CAD build for the part. Positions are in the model's coordinates, mm. A direction names the side the tool comes from. Coordinates: 2 decimals unless noted, no trailing zeros. Order: outer loops, then holes, each group sorted by start corner. A loop starts at its lowest first (then second) coordinate and runs counter-clockwise, first axis right, second up. Notation, with made-up numbers: (54.5, 0.25) - (107.5, 0.25) arc R15 cw to (107.5, 8.25) - close; hole circle Ø10 at (3.5, -28). An arc over 180 degrees is marked (long way). Use one line per item in the form item = value.
```python
from build123d import *

# Parameters (mm, degrees)
F0_R          = 12.7
F1_DEPTH      = 419.1
F0_W          = 165.1
F0_H          = 152.4
F2_DEPTH      = 685.8
F3_DEPTH      = 25.4
F8_DEPTH      = 165.1010001
F8_DEPTH_BACK = 165.1010001
F9_R          = 25.4


with BuildPart() as f1:
    # F0 (on Top) → F1 (new body)
    with BuildSketch(Plane.XY):
        with BuildLine():
            Line((0, -266.7), (0, -152.4))
            Line((0, -152.4), (-165.1, -152.4))
            Line((-165.1, -152.4), (-165.1, -457.2))
            ThreePointArc((-165.1, -457.2), (-116.7433295739, -573.9433295739), (0, -622.3))
            Line((0, -622.3), (0, -342.9))
            ThreePointArc((0, -342.9), (-38.1, -304.8), (0, -266.7))
        make_face()
        with Locations((-101.6, -203.2)):
            Circle(F0_R, mode=Mode.SUBTRACT)
        with Locations((-101.6, -203.2)):
            Circle(F0_R)
        with BuildLine():
            Line((0, -342.9), (0, -266.7))
            ThreePointArc((0, -266.7), (-38.1, -304.8), (0, -342.9))
        make_face()
    extrude(amount=F1_DEPTH)

    # F0 (on Top) → F2 (join)
    with BuildSketch(Plane.XY):
        with Locations((-82.55, -76.2)):
            Rectangle(F0_W, F0_H)
    extrude(amount=F2_DEPTH)

    # F0 (on Top) → F3 (cut)
    with BuildSketch(Plane.XY):
        with BuildLine():
            Line((0, -342.9), (0, -266.7))
            ThreePointArc((0, -266.7), (-38.1, -304.8), (0, -342.9))
        make_face()
    extrude(amount=F3_DEPTH, mode=Mode.SUBTRACT)

    # F4: F1 across face


with BuildPart() as f1_1:
    add(f1.part)
    add(f1.part.mirror(Plane(origin=(0, -279.3076736672, 257.3545234249), x_dir=(0, 1, 0), z_dir=(1, 0, 0))))

    # F6: sweep along a path in F6_path
    with BuildLine(Plane(origin=(-165.1, -152.4, 419.1), x_dir=(0, 1, 0), z_dir=(0, 0, 1))) as f6_path:
        Line((0, 0), (-304.8, 0))
        ThreePointArc((-304.8, 0), (-469.9, -165.1), (-304.8, -330.2))
        Line((-304.8, -330.2), (0, -330.2))
    # F5 (on face) → F6 (sweep, cut)
    with BuildSketch(Plane.XZ.offset(152.4)):
        with BuildLine():
            ThreePointArc((-120.65, 254), (-152.8833058285, 278.74418592), (-165.1, 317.5))
            Line((-165.1, 317.5), (-165.1, 0))
            Line((-165.1, 0), (-139.7, 0))
            Line((-139.7, 0), (-120.65, 254))
        make_face()
    sweep(path=f6_path.line, mode=Mode.SUBTRACT)

    # F7 (on Right) → F8 (cut, two sides)
    with BuildSketch(Plane.YZ) as f8_sk:
        with BuildLine():
            add(Edge.make_bspline(
                [(-76.2, 0), (-76.2, 31.8793983715), (-69.0790448855, 184.3952112859), (-38.761105776, 317.4984685435), (0, 330.2)],
                knots=[0, 0, 0, 0, 0.5205513628, 1, 1, 1, 1], degree=3))
            Line((-76.2, 0), (0, 0))
            Line((0, 0), (0, 330.2))
        make_face()
    extrude(amount=-F8_DEPTH, mode=Mode.SUBTRACT)
    extrude(f8_sk.sketch, amount=F8_DEPTH_BACK, mode=Mode.SUBTRACT)

    # F9
    f9_edges = [f1_1.edges().sort_by_distance(p)[0] for p in [
        (-165.1, -76.2, 685.8),
        (-165.1, -152.4, 552.45),
        (0, -152.4, 685.8),
        (165.1, -76.2, 685.8),
        (165.1, -152.4, 552.45),
        (165.1, -304.8, 419.1),
        (0, -622.3, 419.1),
        (-165.1, -304.8, 419.1),
    ]]
    fillet(f9_edges, radius=F9_R)


solid = f1_1.part
```
Item 1: 3-axis set-ups, long thin cutter, end or side, ignore diameter. For faces 1 (the face through (-130.31, -306.93, 125.22)), 2 (the face through (-157.86, -289.79, 411.46)), 3 (the face through (130.31, -302.67, 125.22)), 4 (the face through (3.63, -622.26, 355.07)), 5 (the face through (-2.86, -587.21, 128.78)): which of +Z, -Z, +X, -X, +Y, -Y reach the whole face in a straight line?
Derived:
face_1 = -X, -Y
face_2 = +Z, -X, -Y
face_3 = +X, -Y
face_4 = +Z, -Z, -Y
face_5 = -Y
Item 2: Drill centre lines: line 1 (Z direction, x = 30.5, y = -408); line 2 (Y direction, x = -141.5, z = 570); line 3 (Y direction, x = 65, z = 643.5). Where is each one in solid material? Low to high. Write a range as [from, to].
Derived:
line_1 = [0, 419.1]
line_2 = [-152.34, 0]
line_3 = [-152.4, 0]
Item 3: Drop flat-ended pins along their axis: pin 1 (19 mm diameter, centred on x = 15.5, y = -320.5, fed in from -Z); pin 2 (8 mm diameter, centred on y = -171, z = 183.5, fed in from +X); pin 3 (2 mm diameter, centred on y = -513.5, z = 172.5, fed in from +X). Give the stop position or say it passes through.
Derived:
pin_1 = 25.4
pin_2 = 126.24
pin_3 = 114.07
Item 4: Two-plate mould, pull along Z, no slides. Class faces 6 (the face through (157.86, -294.41, 411.46)), 7 (the face through (153.2, -302.7, 279.2)), 8 (the face through (-153.2, -306.9, 279.2)), 9 (the face through (2, -152.4, 538)): +Z half, -Z half, draft (parallel to the pull), parting line (faces both ways), or undercut.
Derived:
face_6 = +Z half
face_7 = undercut
face_8 = undercut
face_9 = draft
Item 5: Cut at B-B, the plane z = 581. Write the cut outline in (x, y), plus the area to 3 significant figures.
Derived:
outline = (-165.1, -127) arc R25.4 ccw to (-139.7, -152.4) - (139.7, -152.4) arc R25.4 ccw to (165.1, -127) - (165.1, 0) - (-165.1, 0) - close
area = 50,000 mm²
Item 6: Cut at C-C, the plane y = -391. Write the cut outline in (x, z).
Derived:
outline = (-165.1, 317.5) arc R67.58 ccw to (-120.65, 254) - (-139.7, 0) - (139.7, 0) - (120.65, 254) arc R67.58 ccw to (165.1, 317.5) - (165.1, 393.7) arc R25.4 ccw to (139.7, 419.1) - (-139.7, 419.1) arc R25.4 ccw to (-165.1, 393.7) - close
Item 7: Cut at A-A, the plane y = -304.8. Write the cut outline in (x, z).
Derived:
outline = (-165.1, 317.5) arc R67.58 ccw to (-120.65, 254) - (-139.7, 0) - (-38.1, 0) - (-38.1, 25.4) - (38.1, 25.4) - (38.1, 0) - (139.7, 0) - (120.65, 254) arc R67.58 ccw to (165.1, 317.5) - (165.1, 393.7) arc R25.4 ccw to (139.7, 419.1) - (-139.7, 419.1) arc R25.4 ccw to (-165.1, 393.7) - close
